from build123d import *

# Parameters (mm, degrees)
SKETCH1_W                                            = 60
SKETCH1_H                                            = 60
BOSS_EXTRUDE1_DEPTH                                  = 8
M8_CLEARANCE_HOLE1_D                                 = 9
F_3_0MM_DOWEL_HOLE1_D                                = 3
CBORE_FOR_M3_HEX_SOCKET_THIN_HEAD_CAP_SC_D           = 3.4
CBORE_FOR_M3_HEX_SOCKET_THIN_HEAD_CAP_SC_CBORE_D     = 6.5
CBORE_FOR_M3_HEX_SOCKET_THIN_HEAD_CAP_SC_CBORE_DEPTH = 2.4


with BuildPart() as part:
    # Sketch1 → Boss-Extrude1 (new body)
    with BuildSketch(Plane.XY):
        with Locations((30, 30)):
            Rectangle(SKETCH1_W, SKETCH1_H)
    extrude(amount=BOSS_EXTRUDE1_DEPTH)

    # M8 Clearance Hole1 (through all)
    with Locations(Plane.XY.offset(8)):
        with Locations((30, 30)):
            Hole(M8_CLEARANCE_HOLE1_D / 2)

    # Ø3.0mm Dowel Hole1 (through all)
    with Locations(Plane.XY.offset(8)):
        with Locations((19.607695155, 24), (30, 42), (40.392304845, 24)):
            Hole(F_3_0MM_DOWEL_HOLE1_D / 2)

    # CBORE for M3 Hex Socket Thin Head Cap Screw1 (through all)
    with Locations(Plane.XY.offset(8)):
        with Locations((40.392304845, 36), (30, 18), (19.607695155, 36)):
            CounterBoreHole(CBORE_FOR_M3_HEX_SOCKET_THIN_HEAD_CAP_SC_D / 2, CBORE_FOR_M3_HEX_SOCKET_THIN_HEAD_CAP_SC_CBORE_D / 2, CBORE_FOR_M3_HEX_SOCKET_THIN_HEAD_CAP_SC_CBORE_DEPTH)


solid = part.part
Design review of the part built by this model. Coordinates are the model's own, in mm. A direction names the side the tool comes from. Give positions to 0.01 mm unless a question says otherwise; leave off trailing zeros. Loops run counter-clockwise (first coordinate to the right, second up) from the corner with the lowest first, then second, coordinate; pieces in that order, holes last. Notation, with made-up numbers: M 57.5,-26.5 L 84.5,-26.5 A20 cw 84.5,-2.5 Z; hole C -38,87 d4. An arc over 180 degrees is marked long. One line per question, with ' | ' between items. Start each with the question number.
1. To check wall thickness, follow L1, parallel to Y at x = 30, z = 5.25; L2, parallel to X at y = 38, z = 6.5; L3, parallel to Y at x = 32, z = 6.75. State the ranges of each line that lie inside material, in increasing order.
2. Add section A-A (y = 42). Write out the cut boundary in (x, z).
3. Add section D-D (y = 36). Write out the cut boundary in (x, z).
4. Add section C-C (z = 7). Write out the cut boundary in (x, y), plus the area to 3 significant figures.
5. For faces 4 (the face through (30, 60, 4)), 5 (the face through (37.813, 34.022, 6.817)), list the 3-axis set-ups (+Z, -Z, +X, -X, +Y, -Y) from which the entire face can be reached by the end or side of a thin tool; tool diameter is ignored.
6. The part is to be moulded in two halves that separate along Y. For faces 1 (the face through (41.5, 25.01, 3.94)), 2 (the face through (30, 37, 0)), 3 (the face through (30, 0, 4)), say which applies: released by +Y, released by -Y, zero draft, split by the parting line, or undercut.
7. Insertion check: P1, Ø3, axis at x = 18, y = 36.5, coming from the +Z side; P2, Ø2, axis at x = 30, y = 18, coming from the +Z side. Each pin has a flat end and moves straight along its axis. Give the tip position at first contact, or say it passes through.
8. Add section B-B (x = 30). Write out the cut boundary in (y, z), plus the area to 3 significant figures.
Worked out:
1) L1: y = 0 to 16.3, 19.7 to 25.5, 34.5 to 40.5, 43.5 to 60 | L2: x = 0 to 17.05, 22.17 to 37.83, 42.95 to 60 | L3: y = 0 to 15.44, 20.56 to 25.97, 34.03 to 60
2) outline: M 0,0 L 28.5,0 L 28.5,8 L 0,8 Z; M 31.5,0 L 60,0 L 60,8 L 31.5,8 Z
3) outline: M 0,0 L 17.91,0 L 17.91,5.6 L 16.36,5.6 L 16.36,8 L 0,8 Z; M 21.31,0 L 38.69,0 L 38.69,5.6 L 37.14,5.6 L 37.14,8 L 22.86,8 L 22.86,5.6 L 21.31,5.6 Z; M 42.09,0 L 60,0 L 60,8 L 43.64,8 L 43.64,5.6 L 42.09,5.6 Z
4) outline: M 0,0 L 60,0 L 60,60 L 0,60 Z; hole C 19.61,36 d6.5; hole C 19.61,24 d3; hole C 30,30 d9; hole C 30,18 d6.5; hole C 30,42 d3; hole C 40.39,36 d6.5; hole C 40.39,24 d3 | area: 3,420 mm²
5) face 4: +Z, -Z, +X, -X, +Y | face 5: +Z
6) face 1: undercut | face 2: zero draft | face 3: released by -Y
7) P1: stops at z = 5.6 | P2: passes through
8) outline: M 0,0 L 16.3,0 L 16.3,5.6 L 14.75,5.6 L 14.75,8 L 0,8 Z; M 19.7,0 L 25.5,0 L 25.5,8 L 21.25,8 L 21.25,5.6 L 19.7,5.6 Z; M 34.5,0 L 40.5,0 L 40.5,8 L 34.5,8 Z; M 43.5,0 L 60,0 L 60,8 L 43.5,8 Z | area: 349 mm²
